Could you check a few things on this model? Use its own coordinates, in mm. A direction names the side the tool comes from. Round coordinates to 2 decimals unless told otherwise and drop trailing zeros. Write each loop counter-clockwise with the first axis right and the second up, starting at its lowest first coordinate (ties: lowest second). Pieces come first, ordered by that corner, then holes. Notation, with made-up numbers: (8.5, 89.25) -> (25.5, 89.25) arc R26 ccw to (25.5, 120.25) -> close; hole circle Ø9 at (76.25, -10.5). An arc over 180 degrees is marked (long way). Answer as CSV lines item,"result". Start each with the question number.
Q1. Imagine slicing it at B-B on z = -26. Please give me the cut outline in (x, y) (1 decimal), and give its area (3 significant figures).
Q2. If we mould it in two halves opening along X, with no side actions, what happens to faces 3 (the flat face through (0, 3.572, -7)), 4 (the flat face through (0, 0, 27.75)), 5 (the cylindrical face through (0, -4, 24))? For each: pulls with the +X half, pulls with the -X half, needs draft (parallel to the pull), parting line crosses it, or undercut.
Q3. Imagine slicing it at A-A on x = 0. Please give me the cut outline in (y, z).
Q4. For faces 1 (the flat face through (0.3, -4.4, 19.75)), 2 (the flat face through (0, 0, -41.076)), which set-ups out of +Z, -Z, +X, -X, +Y, -Y let a thin tool reach every point of the face, with its end or its side?
Q5. If I drill on line 1 (X direction, y = 4, z = -14.5); line 2 (X direction, y = -3, z = -2); line 3 (X direction, y = 0.25, z = 0.5), over which ranges is the centre line in solid material (lowest first)? Write a range as [from, to].
Q6. Will these pins go through, and if not, where does the flat tip stop? pin 1 Ø1 at (y, z) = (1.5, 3.5) entering from +X; pin 2 Ø1.1 at (y, z) = (4, -10) entering from -X; pin 3 Ø5 at (y, z) = (-3.5, -15.5) entering from -X.
from build123d import *
from OCP.BRepFilletAPI import BRepFilletAPI_MakeChamfer

# Parameters (mm, degrees)
BOSS_EXTRUDE1_DEPTH      = 27.750000126
BOSS_EXTRUDE1_DEPTH_BACK = 41.075600094
SKETCH5_R                = 4.7625
SKETCH5_R_2              = 4
CUT_EXTRUDE1_DEPTH       = 8
CHAMFER1_SIZE            = 0.47625
CHAMFER1_SIZE2           = 0.173340824
FILLET1_R                = 0.254


with BuildPart() as part:
    # Sketch3 → Boss-Extrude1 (new, two sides: drawn at the far end of the back side and taken through both)
    with BuildSketch(Plane.XY.offset(-BOSS_EXTRUDE1_DEPTH_BACK)):
        with BuildLine():
            Line((-1.1938, 3.571875), (-1.1938, 4.610449849))
            ThreePointArc((-1.1938, 4.610449849), (-2.915127249, -3.766090728), (4.7625, 0))
            ThreePointArc((4.7625, 0), (3.766090728, 2.915127249), (1.1938, 4.610449849))
            Line((1.1938, 4.610449849), (1.1938, 3.571875))
            Line((1.1938, 3.571875), (-1.1938, 3.571875))
        make_face()
    extrude(amount=BOSS_EXTRUDE1_DEPTH + BOSS_EXTRUDE1_DEPTH_BACK)

    # Sketch5 → Cut-Extrude1 (cut)
    with BuildSketch(Plane.XY.offset(27.750000126)):
        Circle(SKETCH5_R)
        Circle(SKETCH5_R_2, mode=Mode.SUBTRACT)
    extrude(amount=-CUT_EXTRUDE1_DEPTH, mode=Mode.SUBTRACT)

    # Chamfer1: one chamfer whose edges measure the first distance from different faces: ONE call of the kernel's chamfer builder (chamfer() names one face for all edges)
    chamfer1_edges_1 = [part.edges().sort_by_distance(p)[0] for p in [
        (0, -4, 27.750000126),
    ]]
    chamfer1_side_1 = [part.faces().sort_by_distance(p)[0] for p in [
        (0, -4, 23.750000126),
    ]]
    chamfer1_edges_2 = [part.edges().sort_by_distance(p)[0] for p in [
        (-2.915127249, -3.766090728, 19.750000126),
    ]]
    chamfer1_side_2 = [part.faces().sort_by_distance(p)[0] for p in [
        (-2.915127249, -3.766090728, -10.662799984),
    ]]
    chamfer1_edges_3 = [part.edges().sort_by_distance(p)[0] for p in [
        (-2.915127249, -3.766090728, -41.075600094),
    ]]
    chamfer1_side_3 = [part.faces().sort_by_distance(p)[0] for p in [
        (0, -0.164578508, -41.075600094),
    ]]
    chamfer1 = BRepFilletAPI_MakeChamfer(part.part.solid().wrapped)
    for e in chamfer1_edges_1:
        chamfer1.Add(CHAMFER1_SIZE, CHAMFER1_SIZE2, e.wrapped, chamfer1_side_1[0].wrapped)  # the first distance lies on this face
    for e in chamfer1_edges_2:
        chamfer1.Add(CHAMFER1_SIZE, CHAMFER1_SIZE2, e.wrapped, chamfer1_side_2[0].wrapped)  # the first distance lies on this face
    for e in chamfer1_edges_3:
        chamfer1.Add(CHAMFER1_SIZE, CHAMFER1_SIZE2, e.wrapped, chamfer1_side_3[0].wrapped)  # the first distance lies on this face
    add(Compound.cast(chamfer1.Shape()), mode=Mode.REPLACE)

    # Fillet1
    fillet1_edges = [part.edges().sort_by_distance(p)[0] for p in [
        (0, -4, 19.750000126),
    ]]
    fillet(fillet1_edges, radius=FILLET1_R)


solid = part.part
Checks:
1,outline,"(-1.2, 3.6) -> (-1.2, 4.6) arc R4.8 ccw (long way) to (1.2, 4.6) -> (1.2, 3.6) -> close"
1,area,"68.5 mm^2"
2,face 3,"undercut"
2,face 4,"needs draft"
2,face 5,"parting line crosses it"
3,outline,"(-4.76, -40.9) -> (-4.29, -41.08) -> (3.57, -41.08) -> (3.57, 27.75) -> (-3.83, 27.75) -> (-4, 27.27) -> (-4, 20) arc R0.25 cw to (-4.25, 19.75) -> (-4.59, 19.75) -> (-4.76, 19.27) -> close"
4,face 1,"+Z"
4,face 2,"-Z, +X, -X, +Y, -Y"
5,line 1,"[-2.58, -1.19], [1.19, 2.58]"
5,line 2,"[-3.7, 3.7]"
5,line 3,"[-4.76, 4.76]"
6,pin 1,"x = 4.66"
6,pin 2,"x = -3.28"
6,pin 3,"x = -4.66"
